Design review of the part built by this model. Coordinates are the model's own, in mm. Face numbers are marked on the shaded views. A direction names the side the tool comes from. Round coordinates to 2 decimals unless told otherwise and drop trailing zeros. Write each loop counter-clockwise with the first axis right and the second up, starting at its lowest first coordinate (ties: lowest second). Pieces come first, ordered by that corner, then holes. Notation, with made-up numbers: (81.25, 46.25) -> (92.25, 46.25) arc R9 cw to (92.25, 56.25) -> close; hole circle Ø11 at (41.5, -27). An arc over 180 degrees is marked (long way). Write item = value, one per line. Start each with the question number.
Item 1: Add section D-D, the plane x = 75. State the section outline as (y, z) points, then the cut area to 3 significant figures.
Item 2: For pin 1 Ø11.5 at (x, y) = (15, 12.5) entering from -Z; pin 2 Ø21 at (x, z) = (314.5, -41.5) entering from -Y; pin 3 Ø12 at (y, z) = (126, -44.5) entering from +X, all flat-tipped, find the tip position at first contact; note any pin that passes through.
Item 3: Add section A-A, the plane y = 12.5. State the section outline as (x, z) points, then the cut area to 3 significant figures.
Item 4: To check wall thickness, follow L1, parallel to X at y = 12, z = 2; L2, parallel to Z at x = 201, y = 85.5; L3, parallel to Y at x = 15, z = 1.1. State the ranges of each line that lie inside material, in increasing order.
Item 5: Add section B-B, the plane x = 115. State the section outline as (y, z) points.
Item 6: Machinability: for the marked faces 1 and 2, which of the approach directions +Z, -Z, +X, -X, +Y, -Y give a long, thin tool a straight path to every point of the face, cutting with its end or side? Answer none if there is none.
Item 7: Add section C-C, the plane z = -36.5. State the section outline as (x, y) points, then the cut area to 3 significant figures.
Autodesk Inventor part; units mm, degrees
ref_plane "YZ Plane" through (0, 0, 0) normal (1, 0, 0) x (0, 1, 0)
ref_plane "XZ Plane" through (0, 0, 0) normal (0, 1, 0) x (-1, 0, 0)
ref_plane "XY Plane" through (0, 0, 0) normal (0, 0, 1) x (1, 0, 0)
sketch "草圖1" plane through (0, 0, 0) normal (0, 0, 1) x (1, 0, 0)
  line L0 (0, 0) -> (-7.8042, 0) construction
  line L1 (0, 0) -> (0, -16.694) construction
  line L2 (0, 0) -> (0, 26)
  line L3 (310, 145) -> (310, 102)
  line L4 (130, 18.5892) -> (130, 0)
  line L5 (130, 0) -> (0, 0)
  line L6 (310, 145) -> (368, 145)
  line L7 (375, 138) -> (375, 109)
  line L8 (368, 102) -> (310, 102)
  line L9 (332, 127.5) -> (354, 127.5)
  arc A0 (354, 119.5) -> (354, 127.5) centre (354, 123.5) ccw
  line L10 (354, 119.5) -> (332, 119.5)
  arc A1 (332, 127.5) -> (332, 119.5) centre (332, 123.5) ccw
  circle A2 centre (15, 12.5) radius 4.5
  circle A3 centre (115, 12.5) radius 4.5
  line L11 (15, 12.5) -> (115, 12.5) construction
  arc A4 (10.0507, 40.16) -> (0, 26) centre (15, 26) ccw
  line L12 (9.9762, 40.1337) -> (303.3752, 144.4225)
  line L13 (306.7244, 145) -> (310, 145)
  line L14 (310, 102) -> (305, 102)
  line L15 (291.9625, 109.2052) -> (135.372, 27.4539)
  arc A5 (375, 138) -> (368, 145) centre (368, 138) ccw
  arc A6 (368, 102) -> (375, 109) centre (368, 109) ccw
  arc A7 (302.0606, 104.4) -> (305, 102) centre (305, 105) ccw
  arc A8 (302.0606, 104.4) -> (291.9625, 109.2052) centre (295.202, 103) ccw
  arc A9 (306.7244, 145) -> (303.3752, 144.4225) centre (306.7244, 135) ccw
  arc A10 (135.372, 27.4539) -> (130, 18.5892) centre (140, 18.5892) ccw
  point P0 (130, 34.6822)
  point P1 (375, 145)
  point P2 (375, 102)
  point P3 (65, 12.5)
  point P4 (65, 0)
  point P5 (130, 24.6493)
  point P6 (305, 145)
  point P7 (305, 102)
  point P8 (305, 116.0118)
  dimension "d0" = 130
  dimension "d1" = 145
  dimension "d2" = 43
  dimension "d3" = 65
  dimension "d4" = 8
  dimension "d5" = 30
  dimension "d7" = 18
  dimension "d8" = 310
  dimension "d14" = 12.5
  dimension "d15" = 100
  dimension "d16" = 9
  dimension "d17" = 21.5
  dimension "d20" = 15
  dimension "d21" = 26
  dimension "d23" = 5
  dimension "d24" = 7
  dimension "d26" = 3
  dimension "d28" = 35
  dimension "d29" = 7
  dimension "d30" = 5
  dimension "d31" = 10
  dimension "d32" = 10
  dimension "d33" = 8
extrude "擠出1" add sketch "草圖1" along normal blind 3.5
bend part "折彎零件1" radius 0.5 angle 80 line through (310, 145, 0) along (0, -1, 0) centre toward (0, 0, -1) moving side (1, 0, 0) both sides no
properties part number "0 零件"
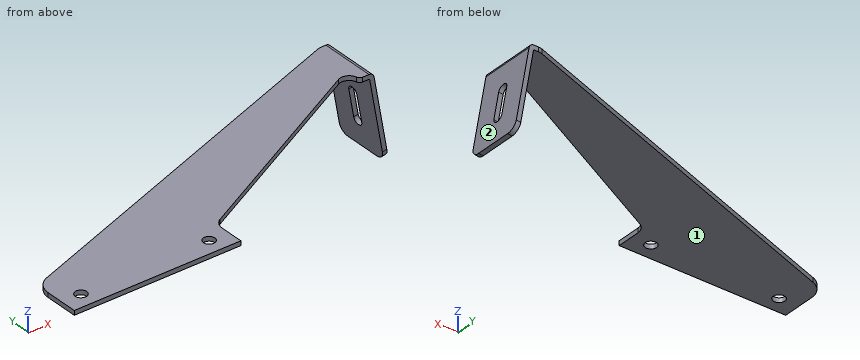
Result set:
q1.outline = (0, 0) -> (63.25, 0) -> (63.25, 3.5) -> (0, 3.5) -> close
q1.area = 221 mm²
q2.pin_1 = 0
q2.pin_2 = 102
q2.pin_3 = 322.88
q3.outline = (0, 0) -> (10.5, 0) -> (10.5, 3.5) -> (0, 3.5) -> close; (19.5, 0) -> (110.5, 0) -> (110.5, 3.5) -> (19.5, 3.5) -> close; (119.5, 0) -> (130, 0) -> (130, 3.5) -> (119.5, 3.5) -> close
q3.area = 392 mm²
q4.L1 = 0 to 10.53, 19.47 to 110.53, 119.47 to 130
q4.L2 = 0 to 3.5
q4.L3 = 0 to 8, 17 to 41.92
q5.outline = (0, 0) -> (8, 0) -> (8, 3.5) -> (0, 3.5) -> close; (17, 0) -> (77.46, 0) -> (77.46, 3.5) -> (17, 3.5) -> close
q6.face_1 = -Z, -X, +Y, -Y
q6.face_2 = +Z, +X, +Y, -Y
q7.outline = (316.86, 102) -> (320.41, 102) -> (320.41, 119.5) -> (316.86, 119.5) -> close; (316.86, 127.5) -> (320.41, 127.5) -> (320.41, 145) -> (316.86, 145) -> close
q7.area = 124 mm²
